```python
from build123d import *

# Parameters (mm, degrees)
F0_R     = 6
F0_R_2   = 2.05
F1_DEPTH = 7
F3_DEPTH = 7.001
F4_R     = 1.1
F5_DEPTH = 4


with BuildPart() as f1:
    # F0 (on Top) → F1 (new body)
    with BuildSketch(Plane.XY):
        Circle(F0_R)
        Circle(F0_R_2, mode=Mode.SUBTRACT)
    extrude(amount=F1_DEPTH)

    # F2 (on face) → F3 (cut, through all)
    with BuildSketch(Plane.XY.offset(7)):
        with BuildLine():
            ThreePointArc((3.490318, 4.880336), (0, 6), (-3.490318, 4.880336))
            Line((-3.490318, 4.880336), (3.490318, 4.880336))
        make_face()
    extrude(amount=-F3_DEPTH, mode=Mode.SUBTRACT)

    # F4 (on face) → F5 (cut)
    with BuildSketch(Plane(origin=(0, 4.880336, 0), x_dir=(-1, 0, 0), z_dir=(0, 1, 0))):
        with Locations((0, 3.5)):
            Circle(F4_R)
    extrude(amount=-F5_DEPTH, mode=Mode.SUBTRACT)


solid = f1.part
```
Verification items for the finished model (mm, model axes). Give positions to 0.01 mm unless a question says otherwise; leave off trailing zeros. Order: outer loops, then holes, each group sorted by start corner. A loop starts at its lowest first (then second) coordinate and runs counter-clockwise, first axis right, second up. Notation, with made-up numbers: (6.25, 10) -> (36.25, 10) arc R24 cw to (36.25, 31) -> close; hole circle Ø7 at (85, 78). An arc over 180 degrees is marked (long way). One line per item, written item: value.
(1) Gauge pin test, flat ends, axial feed: pin 1 (4.5 mm diameter, centred on x = 0, y = 0, fed in from -Z); pin 2 (2 mm diameter, centred on y = -4.5, z = 3, fed in from -X); pin 3 (1.5 mm diameter, centred on x = 4, z = 5, fed in from -Y). Record the tip position at first contact, or that the pin passes through.
Final values:
pin 1: z = 0
pin 2: x = -4.87
pin 3: y = -5.04
(2) Sectioned sample at C-C on z = 0.75. Record the cut outline in (x, y), then the cut area to 3 significant figures.
Final values:
outline: (-3.49, 4.88) arc R6 ccw (long way) to (3.49, 4.88) -> close; hole circle Ø4.1 at (0, 0)
area: 94.6 mm^2
(3) Sectioned sample at A-A on y = 0. Record the cut outline in (x, z), then the cut area to 3 significant figures.
Final values:
outline: (-6, 0) -> (-2.05, 0) -> (-2.05, 7) -> (-6, 7) -> close; (2.05, 0) -> (6, 0) -> (6, 7) -> (2.05, 7) -> close
area: 55.3 mm^2
(4) Draft check along Z on faces 1 (the face through (1.1, 3.3, 3.5)), 2 (the face through (-2, 4.88, 4)), 3 (the face through (1, -2, 0)). Enter one of: pulls with the +Z half, pulls with the -Z half, needs draft (parallel to the pull), parting line crosses it, or undercut.
Final values:
face 1: undercut
face 2: needs draft
face 3: pulls with the -Z half
(5) Sectioned sample at B-B on x = 0. Record the cut outline in (y, z).
Final values:
outline: (-6, 0) -> (-2.05, 0) -> (-2.05, 7) -> (-6, 7) -> close; (2.05, 0) -> (4.88, 0) -> (4.88, 2.4) -> (2.05, 2.4) -> close; (2.05, 4.6) -> (4.88, 4.6) -> (4.88, 7) -> (2.05, 7) -> close
(6) Scan lines: line 1 along Y through (x, z) = (0, 5.5); line 2 along Z through (x, y) = (0, 2.4); line 3 along Y through (x, z) = (-1.5, 2.75). Record each from-to range of solid material in increasing order. Write a range as [from, to].
Final values:
line 1: [-6, -2.05], [2.05, 4.88]
line 2: [0, 2.4], [4.6, 7]
line 3: [-5.81, -1.4], [1.4, 4.88]
(7) Sectioned sample at D-D on z = 3.5. Record the cut outline in (x, y).
Final values:
outline: (-3.49, 4.88) arc R6 ccw (long way) to (3.49, 4.88) -> (1.1, 4.88) -> (1.1, 1.73) arc R2.05 cw (long way) to (-1.1, 1.73) -> (-1.1, 4.88) -> close
